Verification items for the finished model (mm, model axes). Give positions to 0.01 mm unless a question says otherwise; leave off trailing zeros. Write each loop counter-clockwise with the first axis right and the second up, starting at its lowest first coordinate (ties: lowest second). Pieces come first, ordered by that corner, then holes. Notation, with made-up numbers: (82.5, -28) -> (127.5, -28) arc R21 cw to (127.5, 10) -> close; hole circle Ø6 at (85, 45). An arc over 180 degrees is marked (long way). Use one line per item in the form item = value. Start each with the question number.
(1) Section check D-D, the plane z = 2.5. State how many separate pieces and enclosed holes the cut face has, plus the area to 3 significant figures.
(2) Scan lines: L1, parallel to Y at x = -95.5, z = 0.55; L2, parallel to Y at x = -22, z = 1.2; L3, parallel to Y at x = -89.5, z = 1.35. Record each from-to range of solid material in increasing order.
(3) Depth check by flat-ended pin: pin 1 Ø6.5 at (x, y) = (-95.5, -6) entering from +Z; pin 2 Ø0.6 at (y, z) = (0.5, 1.5) entering from +X. Enter the tip coordinate at first touch or a pass-through.
(4) Section check B-B, the plane y = 16. Record the cut outline in (x, z), plus the area to 3 significant figures.
(5) Section check A-A, the plane x = 9.5. Record the cut outline in (y, z).
(6) Section check C-C, the plane x = 89.5. Record the cut outline in (y, z).
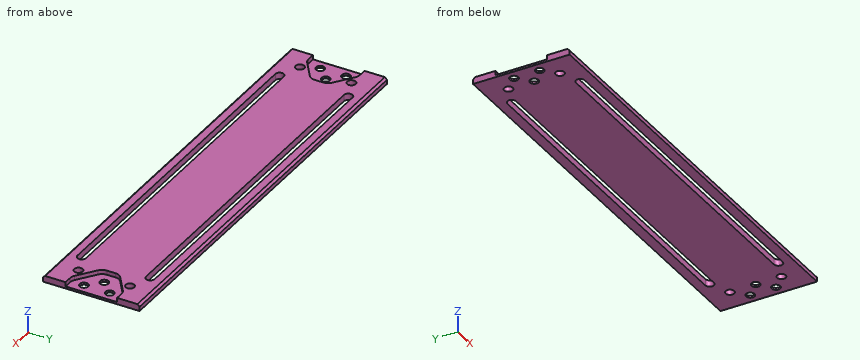
from build123d import *

# Parameters (mm, degrees)
SKETCH1_W            = 200
SKETCH1_H            = 45
BOSS_EXTRUDE1_DEPTH  = 3
SKETCH2_R            = 2
CUT_EXTRUDE1_DEPTH   = 5
CUT_EXTRUDE5_DEPTH   = 2
CHAMFER2_SIZE        = 1
FILLET1_R            = 4
FILLET1_OF_MIRROR4_R = 4
CUT_EXTRUDE6_DEPTH   = 10


with BuildPart() as part:
    # Sketch1 → Boss-Extrude1 (new body)
    with BuildSketch(Plane.XY):
        Rectangle(SKETCH1_W, SKETCH1_H)
    extrude(amount=BOSS_EXTRUDE1_DEPTH)

    # Sketch2 → Cut-Extrude1 (cut)
    with BuildSketch(Plane(origin=(0, 0, 0), x_dir=(-1, 0, 0), z_dir=(0, 0, -1))):
        with Locations((89.5, 0)):
            Circle(SKETCH2_R)
        with Locations((95.5, 6)):
            Circle(SKETCH2_R)
        with Locations((95.5, -6)):
            Circle(SKETCH2_R)
        with Locations((89.5, -12)):
            Circle(SKETCH2_R)
        with Locations((89.5, 12)):
            Circle(SKETCH2_R)
    cut_extrude1 = extrude(amount=-CUT_EXTRUDE1_DEPTH, mode=Mode.SUBTRACT)

    # Sketch8 → Cut-Extrude5 (cut)
    with BuildSketch(Plane.XY.offset(3)):
        Polygon((-84, 4), (-84, -4), (-95, -12), (-100, -12), (-100, 12), (-95, 12), align=None)
    cut_extrude5 = extrude(amount=-CUT_EXTRUDE5_DEPTH, mode=Mode.SUBTRACT)

    # Chamfer2
    chamfer2_edges = [part.edges().sort_by_distance(p)[0] for p in [
        (0, -22.5, 3),
        (0, 22.5, 3),
    ]]
    chamfer(chamfer2_edges, length=CHAMFER2_SIZE)

    # Fillet1
    fillet1_edges = [part.edges().sort_by_distance(p)[0] for p in [
        (-95, 12, 2),
        (-84, 4, 2),
        (-84, -4, 2),
        (-95, -12, 2),
    ]]
    fillet(fillet1_edges, radius=FILLET1_R)

    # Mirror4: Cut-Extrude1, Cut-Extrude5 across plane
    add(cut_extrude1.mirror(Plane(origin=(0, 0, 0), x_dir=(0, 0, 1), z_dir=(1, 0, 0))), mode=Mode.SUBTRACT)
    add(cut_extrude5.mirror(Plane(origin=(0, 0, 0), x_dir=(0, 0, 1), z_dir=(1, 0, 0))), mode=Mode.SUBTRACT)

    # Fillet1 of Mirror4
    fillet1_of_mirror4_edges = [part.edges().sort_by_distance(p)[0] for p in [
        (95, 12, 2),
        (84, 4, 2),
        (84, -4, 2),
        (95, -12, 2),
    ]]
    fillet(fillet1_of_mirror4_edges, radius=FILLET1_OF_MIRROR4_R)

    # Sketch9 → Cut-Extrude6 (cut)
    with BuildSketch(Plane.XY.offset(3)):
        with BuildLine():
            Line((80, -18), (-80, -18))
            ThreePointArc((-80, -18), (-82, -16), (-80, -14))
            Line((-80, -14), (80, -14))
            ThreePointArc((80, -14), (82, -16), (80, -18))
        make_face()
    cut_extrude6 = extrude(amount=-CUT_EXTRUDE6_DEPTH, mode=Mode.SUBTRACT)

    # Mirror5: Cut-Extrude6 across plane
    add(cut_extrude6.mirror(Plane.ZX), mode=Mode.SUBTRACT)


solid = part.part
Completed:
q1.separate_pieces = 1
q1.enclosed_holes = 6
q1.area = 6,860 mm²
q2.L1 = -22.5 to -8, -4 to 4, 8 to 22.5
q2.L2 = -22.5 to -18, -14 to 14, 18 to 22.5
q2.L3 = -22.5 to -14, -10 to -8, 8 to 10, 14 to 22.5
q3.pin_1 = 1
q3.pin_2 = 84
q4.outline = (-100, 0) -> (-82, 0) -> (-82, 3) -> (-100, 3) -> close; (82, 0) -> (100, 0) -> (100, 3) -> (82, 3) -> close
q4.area = 108 mm²
q5.outline = (-22.5, 0) -> (-18, 0) -> (-18, 3) -> (-21.5, 3) -> (-22.5, 2) -> close; (-14, 0) -> (14, 0) -> (14, 3) -> (-14, 3) -> close; (18, 0) -> (22.5, 0) -> (22.5, 2) -> (21.5, 3) -> (18, 3) -> close
q6.outline = (-22.5, 0) -> (-14, 0) -> (-14, 3) -> (-21.5, 3) -> (-22.5, 2) -> close; (-10, 0) -> (-2, 0) -> (-2, 1) -> (-8, 1) -> (-8, 3) -> (-10, 3) -> close; (2, 0) -> (10, 0) -> (10, 3) -> (8, 3) -> (8, 1) -> (2, 1) -> close; (14, 0) -> (22.5, 0) -> (22.5, 2) -> (21.5, 3) -> (14, 3) -> close
